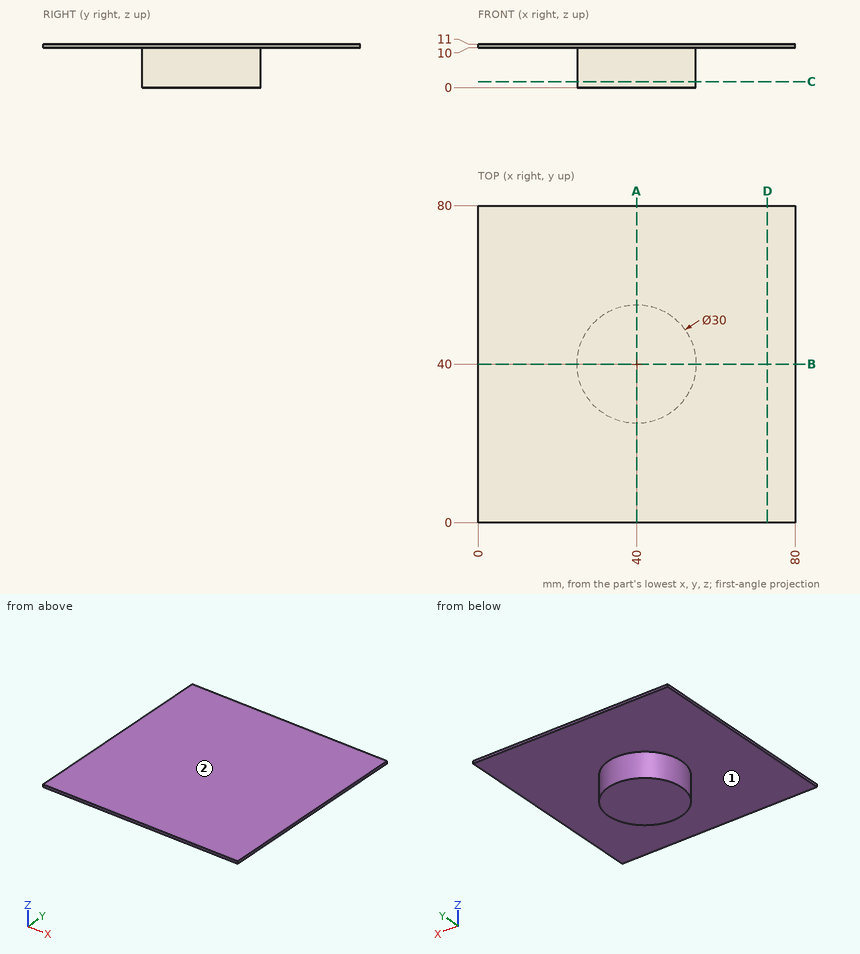
Job drawing, mm, ordinate dimensions from the low corner. One solid piece. A direction names the side the tool comes from. Give positions to 0.01 mm unless a question says otherwise; leave off trailing zeros. Loops run counter-clockwise (first coordinate to the right, second up) from the corner with the lowest first, then second, coordinate; pieces in that order, holes last. Notation, with made-up numbers: M 7,33.5 L 11,33.5 A24 cw 11,48.5 Z; hole C 13,80.25 d9. An arc over 180 degrees is marked long. Use one line per item in the form item = value.
Item 1: Flat gauge pin, fed straight in: pin 1 Ø6 at (x, y) = (30.5, 69) entering from -Z. Where does the tip first touch, or does it go through?
Filled in:
pin_1 = 10
Item 2: Slice it at D-D on x = 73. List the corners of the cut face in (y, z), and give its area (3 significant figures).
Filled in:
outline = M 0,10 L 80,10 L 80,11 L 0,11 Z
area = 80.0 mm^2
Item 3: Slice it at A-A on x = 40. List the corners of the cut face in (y, z).
Filled in:
outline = M 0,10 L 25,10 L 25,0 L 55,0 L 55,10 L 80,10 L 80,11 L 0,11 Z
Item 4: Drill centre lines: L1, parallel to Z at x = 31, y = 62.5; L2, parallel to Y at x = 40, z = 6.25; L3, parallel to X at y = 51.5, z = 1. Where is each one in solid material? Low to high.
Filled in:
L1 = 10 to 11
L2 = 25 to 55
L3 = 30.37 to 49.63
Item 5: Slice it at C-C on z = 1.5. List the corners of the cut face in (x, y).
Filled in:
outline = C 40,40 d30
Item 6: Which spindle directions (+Z, -Z, +X, -X, +Y, -Y) get a long thin tool onto all of the face, cutting with end or side? Do the marked faces 1 and 2. Say none if no direction does.
Filled in:
face_1 = -Z
face_2 = +Z, +X, -X, +Y, -Y
